Input: part model. Units: mm. Frame: model coordinates. Give positions to 0.01 mm unless a question says otherwise; leave off trailing zeros. Order: outer loops, then holes, each group sorted by start corner. A loop starts at its lowest first (then second) coordinate and runs counter-clockwise, first axis right, second up.
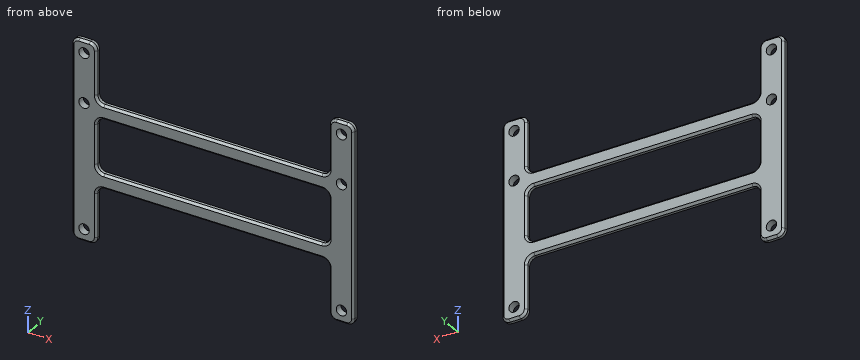
```python
from build123d import *

# Parameters (mm, degrees)
F0_W     = 0.0285906434
F0_H     = 5
F0_W_2   = 40.2
F0_R     = 1.8
F1_DEPTH = 2.5
F2_R     = 2.5
F3_SIZE  = 0.75


# Not quite as in the source:
# - a feature names something its author has since deleted; it is built from what else it names


with BuildPart() as f1:
    # F0 (on Front) → F1 (new body)
    with BuildSketch(Plane.XZ):
        with Locations((-40.2142953217, 18.525)):
            Rectangle(F0_W, F0_H)
        with Locations((40.2142953217, 18.525)):
            Rectangle(F0_W, F0_H)
        with Locations((-20.1, 18.525)):
            Rectangle(F0_W_2, F0_H)
        with Locations((20.1, 18.525)):
            Rectangle(F0_W_2, F0_H)
        with Locations((20.1, 42.125)):
            Rectangle(F0_W_2, F0_H)
        Polygon((40.2, 64.625), (40.2, 44.625), (40.2, 39.625), (40.2, 21.025), (40.2285906434, 21.025), (40.2285906434, 16.025), (40.2, 16.025), (40.2, -3.975), (48.8, -3.975), (48.8, 64.625), align=None)
        with Locations((44.5, 0.325)):
            Circle(F0_R, mode=Mode.SUBTRACT)
        with Locations((44.5, 43.325)):
            Circle(F0_R, mode=Mode.SUBTRACT)
        with Locations((44.5, 60.325)):
            Circle(F0_R, mode=Mode.SUBTRACT)
        with Locations((-20.1, 42.125)):
            Rectangle(F0_W_2, F0_H)
        Polygon((-40.2, 64.625), (-48.8, 64.625), (-48.8, -3.975), (-40.2, -3.975), (-40.2, 16.025), (-40.2285906434, 16.025), (-40.2285906434, 21.025), (-40.2, 21.025), (-40.2, 39.625), (-40.2, 44.625), align=None)
        with Locations((-44.5, 0.325)):
            Circle(F0_R, mode=Mode.SUBTRACT)
        with Locations((-44.5, 43.325)):
            Circle(F0_R, mode=Mode.SUBTRACT)
        with Locations((-44.5, 60.325)):
            Circle(F0_R, mode=Mode.SUBTRACT)
    extrude(amount=F1_DEPTH)

    # F2
    f2_edges = [f1.edges().sort_by_distance(p)[0] for p in [
        (-40.2, -1.25, 44.625),
        (40.2, -1.25, 44.625),
        (-40.2, -1.25, 39.625),
        (40.2, -1.25, 39.625),
        (-40.2, -1.25, 21.025),
        (40.2, -1.25, 21.025),
        (-40.2, -1.25, 16.025),
        (40.2, -1.25, 16.025),
        (40.2, -1.25, -3.975),
        (48.8, -1.25, -3.975),
        (-48.8, -1.25, -3.975),
        (-40.2, -1.25, -3.975),
        (48.8, -1.25, 64.625),
        (40.2, -1.25, 64.625),
        (-48.8, -1.25, 64.625),
        (-40.2, -1.25, 64.625),
    ]]
    fillet(f2_edges, radius=F2_R)

    # F3
    f3_edges = [f1.edges().sort_by_distance(p)[0] for p in [
        (0, 0, 16.025),
        (0, 0, 39.625),
        (-44.5, -2.5, 64.625),
        (0, -2.5, 39.625),
    ]]
    chamfer(f3_edges, length=F3_SIZE)


solid = f1.part
```
1) First-contact query: P1, Ø5, axis at x = -38.5, z = 53.5, coming from the -Y side; P2, Ø0.8, axis at x = -11.5, y = -1.5, coming from the +Z side (3 decimals); P3, Ø0.8, axis at x = 7, y = -1.5, coming from the -Z side (3 decimals). Flat tips, straight axial feed; report the tip coordinate or a pass-through.
2) Cut plane B-B (x = 16). Return the cut outline in (y, z) (3 decimals).
3) Line query: probe 1 along Z at (x, y) = (44.5, -1.55) (3 decimals); probe 2 along X at (y, z) = (-0.9, 61); probe 3 along Z at (x, y) = (-24.5, -1.35) (3 decimals). Output: solid intervals per line, ascending.
4) Cut plane A-A (z = 33). Return the cut outline in (x, y).
5) Cut plane C-C (x = -44.5). Return the cut outline in (y, z) (3 decimals).
Geometry says:
1. P1: stops at y = -2.5
1. P2: stops at z = 44.625
1. P3: stops at z = 16.025
2. outline: (-2.5, 16.775) - (-1.75, 16.025) - (-0.75, 16.025) - (0, 16.775) - (0, 20.275) - (-0.75, 21.025) - (-1.75, 21.025) - (-2.5, 20.275) - close; (-2.5, 40.375) - (-1.75, 39.625) - (-0.75, 39.625) - (0, 40.375) - (0, 43.875) - (-0.75, 44.625) - (-1.75, 44.625) - (-2.5, 43.875) - close
3. probe 1: z = -3.975 to -1.475, 2.125 to 41.525, 45.125 to 58.525, 62.125 to 64.625
3. probe 2: x = -48.8 to -46.17, -42.83 to -40.2, 40.2 to 42.83, 46.17 to 48.8
3. probe 3: z = 16.025 to 21.025, 39.625 to 44.625
4. outline: (-48.8, -1.75) - (-48.05, -2.5) - (-40.95, -2.5) - (-40.2, -1.75) - (-40.2, -0.75) - (-40.95, 0) - (-48.05, 0) - (-48.8, -0.75) - close; (40.2, -1.75) - (40.95, -2.5) - (48.05, -2.5) - (48.8, -1.75) - (48.8, -0.75) - (48.05, 0) - (40.95, 0) - (40.2, -0.75) - close
5. outline: (-2.5, -3.225) - (-1.75, -3.975) - (-0.75, -3.975) - (0, -3.225) - (0, -1.475) - (-2.5, -1.475) - close; (-2.5, 2.125) - (0, 2.125) - (0, 41.525) - (-2.5, 41.525) - close; (-2.5, 45.125) - (0, 45.125) - (0, 58.525) - (-2.5, 58.525) - close; (-2.5, 62.125) - (0, 62.125) - (0, 63.875) - (-0.75, 64.625) - (-1.75, 64.625) - (-2.5, 63.875) - close
